```python
from build123d import *

# Parameters (mm, degrees)
SKETCH_1_W          = 224
SKETCH_1_H          = 44
EXTRUDE_1_DEPTH     = 10
SKETCH_2_R          = 2.1
SKETCH_2_R_2        = 1.65
CUT_EXTRUDE_1_DEPTH = 121.747670785
EXTRUDE_2_DEPTH     = 10
SKETCH_5_R          = 1.65
CUT_EXTRUDE_2_DEPTH = 10
SKETCH_6_R          = 1.65
CUT_EXTRUDE_3_DEPTH = 116.879247495
FILLET_1_R          = 10
SKETCH_7_W          = 18
SKETCH_7_H          = 34
SKETCH_7_W_2        = 15.25
SKETCH_7_W_3        = 30
CUT_EXTRUDE_4_DEPTH = 116.879247495
FILLET_2_R          = 3


with BuildPart() as part:
    # 草图1 → 凸台-拉伸1 (new body)
    with BuildSketch(Plane.XY):
        Rectangle(SKETCH_1_W, SKETCH_1_H)
    extrude(amount=EXTRUDE_1_DEPTH)

    # 草图2 → 切除-拉伸1 (cut, through all)
    with BuildSketch(Plane(origin=(0, 22, 0), x_dir=(1, 0, 0), z_dir=(0, 1, 0))):
        with Locations(Location((-40, -5, 0), (0, 0, 180))):
            Circle(SKETCH_2_R)
        with Locations(Location((-50, -5, 0), (0, 0, 180))):
            Circle(SKETCH_2_R)
        with Locations((50, -5)):
            Circle(SKETCH_2_R)
        with Locations((40, -5)):
            Circle(SKETCH_2_R)
        with Locations(Location((-15, -5, 0), (0, 0, 180))):
            Circle(SKETCH_2_R_2)
        with Locations((15, -5)):
            Circle(SKETCH_2_R_2)
    extrude(amount=-CUT_EXTRUDE_1_DEPTH, mode=Mode.SUBTRACT)

    # 草图4 → 凸台-拉伸2 (add)
    with BuildSketch(Plane.XY.offset(10)):
        Polygon((112, 22), (112, 28), (104, 28), (87, 22), align=None)
        Polygon((-87, 22), (-112, 22), (-112, 28), (-104, 28), align=None)
    extrude(amount=-EXTRUDE_2_DEPTH)

    # 草图5 → 切除-拉伸2 (cut)
    with BuildSketch(Plane(origin=(112, 0, 0), x_dir=(0, 0, -1), z_dir=(1, 0, 0))):
        with Locations((-5, 23)):
            Circle(SKETCH_5_R)
        with Locations((-5, 13)):
            Circle(SKETCH_5_R)
        with Locations((-5, 3)):
            Circle(SKETCH_5_R)
        with Locations((-5, -7)):
            Circle(SKETCH_5_R)
        with Locations((-5, -17)):
            Circle(SKETCH_5_R)
    cut_extrude_2 = extrude(amount=-CUT_EXTRUDE_2_DEPTH, mode=Mode.SUBTRACT)

    # 镜向1: 切除-拉伸2 across plane
    add(cut_extrude_2.mirror(Plane(origin=(0, 0, 0), x_dir=(0, 0, 1), z_dir=(1, 0, 0))), mode=Mode.SUBTRACT)

    # 草图6 → 切除-拉伸3 (cut, through all)
    with BuildSketch(Plane.XY.offset(10)):
        with Locations((-100, 10)):
            Circle(SKETCH_6_R)
        with Locations((-100, -10)):
            Circle(SKETCH_6_R)
        with Locations(Location((100, -10, 0), (0, 0, 180))):
            Circle(SKETCH_6_R)
        with Locations(Location((100, 10, 0), (0, 0, 180))):
            Circle(SKETCH_6_R)
        with Locations((-90, 10)):
            Circle(SKETCH_6_R)
        with Locations((-90, -10)):
            Circle(SKETCH_6_R)
        with Locations(Location((90, -10, 0), (0, 0, 180))):
            Circle(SKETCH_6_R)
        with Locations(Location((90, 10, 0), (0, 0, 180))):
            Circle(SKETCH_6_R)
    extrude(amount=-CUT_EXTRUDE_3_DEPTH, mode=Mode.SUBTRACT)

    # 圆角1
    fillet_1_edges = [part.edges().sort_by_distance(p)[0] for p in [
        (87, 22, 5),
        (104, 28, 5),
        (-104, 28, 5),
        (-87, 22, 5),
    ]]
    fillet(fillet_1_edges, radius=FILLET_1_R)

    # 草图7 → 切除-拉伸4 (cut, through all)
    with BuildSketch(Plane.XY.offset(10)):
        Rectangle(SKETCH_7_W, SKETCH_7_H)
        with Locations((27.275, 0)):
            Rectangle(SKETCH_7_W_2, SKETCH_7_H)
        with Locations((70.1, 0)):
            Rectangle(SKETCH_7_W_3, SKETCH_7_H)
        with Locations((-70.1, 0)):
            Rectangle(SKETCH_7_W_3, SKETCH_7_H)
        with Locations((-27.275, 0)):
            Rectangle(SKETCH_7_W_2, SKETCH_7_H)
    extrude(amount=-CUT_EXTRUDE_4_DEPTH, mode=Mode.SUBTRACT)

    # 圆角2
    fillet_2_edges = [part.edges().sort_by_distance(p)[0] for p in [
        (-19.65, 17, 5),
        (-19.65, -17, 5),
        (-34.9, -17, 5),
        (-34.9, 17, 5),
        (-85.1, -17, 5),
        (-85.1, 17, 5),
        (-55.1, 17, 5),
        (-55.1, -17, 5),
        (55.1, -17, 5),
        (55.1, 17, 5),
        (85.1, 17, 5),
        (85.1, -17, 5),
        (34.9, 17, 5),
        (34.9, -17, 5),
        (19.65, -17, 5),
        (19.65, 17, 5),
        (9, 17, 5),
        (9, -17, 5),
        (-9, -17, 5),
        (-9, 17, 5),
    ]]
    fillet(fillet_2_edges, radius=FILLET_2_R)


solid = part.part
```
Model file for the job. Use its own axes, mm. A direction names the side the tool comes from. Round coordinates to 2 decimals unless told otherwise and drop trailing zeros. Write each loop counter-clockwise with the first axis right and the second up, starting at its lowest first coordinate (ties: lowest second). Pieces come first, ordered by that corner, then holes. Notation, with made-up numbers: (-24.75, 28) - (30.25, 28) arc R4 cw to (30.25, 33) - close; hole circle Ø10 at (15, 75). An arc over 180 degrees is marked (long way). Use CSV: the item, a comma, the result in double quotes. Start each with the question number.
Item 1: Tool access for faces 4 (the face through (112, 3, 7)), 5 (the face through (-1, 22, 5)), 6 (the face through (55.1, 0, 5)): list every direction of +Z, -Z, +X, -X, +Y, -Y with a clear straight run to the whole face (end or side of a thin tool).
Item 2: Pin check, flat tips, straight feed: P1, Ø1.5, axis at x = -36, z = 5.5, coming from the +Y side; P2, Ø3, axis at x = -100, y = 10, coming from the +Z side; P3, Ø3, axis at y = 13, z = 5, coming from the -X side. Stop position of each tip, or through.
Item 3: Band-saw the part on B-B (y = 19.5). Write the cut outline in (x, z), and give its area (3 significant figures).
Item 4: Band-saw the part on C-C (y = -1). State how many separate pieces and enclosed holes the cut face has, and give its area (3 significant figures).
Item 5: Drill centre lines: L1, parallel to X at y = 3, z = 1.5; L2, parallel to Y at x = -78.5, z = 3; L3, parallel to Y at x = -90, z = 2. Where is each one in solid material? Low to high. Write a range as [from, to].
Item 6: Two-plate mould, pull along Z, no slides. Class faces 1 (the face through (-2, 20, 10)), 2 (the face through (-70, 17, 5)), 3 (the face through (-37.9, 0.31, 5.09)): released by +Z, released by -Z, zero draft, split by the parting line, or undercut.
Item 7: Band-saw the part on A-A (x = 67). Write the cut outline in (y, z), and give its area (3 significant figures).
Item 8: Band-saw the part on D-D (x = -40). Write the cut outline in (y, z), and give its area (3 significant figures).
Checked values:
1,face 4,"+Z, -Z, +X, +Y, -Y"
1,face 5,"+Z, -Z, +Y"
1,face 6,"+Z, -Z"
2,P1,"stops at y = 22"
2,P2,"passes through"
2,P3,"stops at x = -102"
3,outline,"(-112, 0) - (112, 0) - (112, 10) - (-112, 10) - close; hole circle Ø4.2 at (-50, 5); hole circle Ø4.2 at (-40, 5); hole circle Ø3.3 at (-15, 5); hole circle Ø3.3 at (15, 5); hole circle Ø4.2 at (40, 5); hole circle Ø4.2 at (50, 5)"
3,area,"2,170 mm²"
4,separate pieces,"6"
4,enclosed holes,"6"
4,area,"1,080 mm²"
5,L1,"x = [-112, -85.1], [-55.1, -34.9], [-19.65, -9], [9, 19.65], [34.9, 55.1], [85.1, 112]"
5,L2,"y = [-22, -17], [17, 22]"
5,L3,"y = [-22, -11.65], [-8.35, 8.35], [11.65, 23.06]"
6,face 1,"released by +Z"
6,face 2,"zero draft"
6,face 3,"undercut"
7,outline,"(-22, 0) - (-17, 0) - (-17, 10) - (-22, 10) - close; (17, 0) - (22, 0) - (22, 10) - (17, 10) - close"
7,area,"100 mm²"
8,outline,"(-22, 0) - (22, 0) - (22, 2.9) - (-22, 2.9) - close; (-22, 7.1) - (22, 7.1) - (22, 10) - (-22, 10) - close"
8,area,"255 mm²"
